Here's how the part is built. I have some questions about the finished solid (model axes, mm). Face numbers are marked on the shaded views. A direction names the side the tool comes from. Coordinates: 2 decimals unless noted, no trailing zeros. Write each loop counter-clockwise with the first axis right and the second up, starting at its lowest first coordinate (ties: lowest second). Pieces come first, ordered by that corner, then holes. Notation, with made-up numbers: (72, 34.25) -> (117, 34.25) arc R33 ccw to (117, 72.25) -> close; hole circle Ø8 at (36, 0). An arc over 180 degrees is marked (long way). Put each result on its own line as item: value. Start each with the question number.
Item 1: I need wall thicknesses on line 1 (X direction, y = -5, z = -2); line 2 (X direction, y = 11, z = -10); line 3 (X direction, y = -10, z = -11.5). Which ranges of each line are inside material? Lowest first, please. Write a range as [from, to].
Item 2: If we mould it in two halves opening along X, with no side actions, what happens to the marked faces 6, 7, 8 and 9? For each: released by +X, released by -X, zero draft, split by the parting line, or undercut.
Item 3: I want a section at A-A, the plane y = -4. List the corners of the cut face in (x, z) for me, then the cut area to 3 significant figures.
Item 4: I want a section at B-B, the plane z = -11. State how many separate pieces and enclosed holes the cut face has, then the cut area to 3 significant figures.
Item 5: For pin 1 (2 mm diameter, centred on x = -9.5, z = -8.5, fed in from +Y); pin 2 (1 mm diameter, centred on x = -14.5, z = -5.5, fed in from +Y); pin 3 (3.5 mm diameter, centred on y = 13, z = -10.5, fed in from -X), each with a flat end and sliding along its axis, tell me the tip position at first contact or that it passes through.
Item 6: I want a section at C-C, the plane x = -27. List the corners of the cut face in (y, z) for me.
Item 7: On a 3-axis mill with a long thin cutter (end or side, diameter ignored), from which of +Z, -Z, +X, -X, +Y, -Y can I reach the whole of each face in a straight line? I mean the marked faces 1, 2, 3, 4 and 5. Say none if no direction works.
from build123d import *

# Parameters (mm, degrees)
F0_W     = 6.6796690226
F0_H     = 6.4269647701
F0_W_2   = 4.7415380832
F0_H_2   = 6.6773667932
F0_W_3   = 4.3679763669
F0_H_3   = 6.5104326932
F3_DEPTH = 17.91377


# Not quite as in the source:
# - a feature of the source that left no trace in its solid (it failed there, or was rolled back) is left out


with BuildPart() as f3:
    # F0 (on Top) → F3 (new body)
    with BuildSketch(Plane.XY):
        with BuildLine():
            Line((-7.7901906334, 10.6832636405), (-7.7901906334, 8.2267736901))
            Line((-7.7901906334, 8.2267736901), (-7.7901906334, 1.7163409969))
            Line((-7.7901906334, 1.7163409969), (-7.7901906334, -5.3760232519))
            add(Edge.make_bspline(
                [(-7.7901906334, -5.3760232519), (-5.8573922142, -16.4409913238), (6.3671558164, -13.6890839785), (6.6410573199, -5.3240084089)],
                knots=[0, 0, 0, 0, 14.4313416921, 14.4313416921, 14.4313416921, 14.4313416921], degree=3))
            Line((6.6410573199, -5.3240084089), (6.6410573199, 1.7169426428))
            Line((6.6410573199, 1.7169426428), (6.6410573199, 8.1439074129))
            Line((6.6410573199, 8.1439074129), (6.6410573199, 10.5028618127))
            add(Edge.make_bspline(
                [(-7.7901906334, 10.6832636405), (-7.9460730776, 20.2635042254), (6.0135321692, 21.5757451952), (6.6410573199, 10.5028618127)],
                knots=[0, 0, 0, 0, 14.4323754909, 14.4323754909, 14.4323754909, 14.4323754909], degree=3))
        make_face()
        with BuildLine():
            Line((-3.0246356037, 8.227375336), (-3.0246356037, 10.4858698323))
            add(Edge.make_bspline(
                [(-3.0246356037, 10.4858698323), (-2.9879831709, 15.9807316959), (2.4520969018, 14.104841277), (1.7169024795, 10.4636372998)],
                knots=[0, 0, 0, 0, 4.7415902058, 4.7415902058, 4.7415902058, 4.7415902058], degree=3))
            Line((1.7169024795, 10.4636372998), (1.7169024795, 8.227375336))
            Line((1.7169024795, 8.227375336), (1.7169024795, 1.5500085428))
            Line((1.7169024795, 1.5500085428), (1.7169024795, -5.1218802109))
            add(Edge.make_bspline(
                [(-3.0246356037, -5.2313073538), (-2.9015108012, -9.3426071107), (2.1988428198, -8.9745400473), (1.7169024795, -5.1218802109)],
                knots=[0, 0, 0, 0, 4.7428006171, 4.7428006171, 4.7428006171, 4.7428006171], degree=3))
            Line((-3.0246356037, -5.2313073538), (-3.0246356037, 1.5500085428))
            Line((-3.0246356037, 1.5500085428), (-3.0246356037, 8.227375336))
        make_face(mode=Mode.SUBTRACT)
        with BuildLine():
            add(Edge.make_bspline(
                [(-20.5391882093, 13.9101054404), (-15.6776210399, 14.6662937362), (-16.1226423563, 15.8139783774), (-15.4372690351, 17.8214814399)],
                knots=[0, 0, 0, 0, 6.4287200491, 6.4287200491, 6.4287200491, 6.4287200491], degree=3))
            Line((-20.5391882093, 13.9101054404), (-20.5391882093, 10.912990186))
            Line((-20.5391882093, 10.912990186), (-16.858519438, 10.912990186))
            Line((-16.858519438, 10.912990186), (-16.858519438, 8.1935095558))
            Line((-16.858519438, 8.1935095558), (-16.858519438, 1.6338703002))
            Line((-16.858519438, 1.6338703002), (-16.858519438, -11.9715025764))
            Line((-16.858519438, -11.9715025764), (-12.1581670002, -11.9715025764))
            Line((-12.1581670002, -11.9715025764), (-12.1581670002, 1.7163409969))
            Line((-12.1581670002, 1.7163409969), (-12.1581670002, 8.2267736901))
            Line((-12.1581670002, 8.2267736901), (-12.1581670002, 17.8214814399))
            Line((-12.1581670002, 17.8214814399), (-15.4372690351, 17.8214814399))
        make_face()
        with BuildLine():
            Line((13.3207263425, 10.6080584228), (13.3207263425, 8.1439074129))
            Line((13.3207263425, 8.1439074129), (13.3207263425, 1.7169426428))
            Line((13.3207263425, 1.7169426428), (13.3207263425, -11.9709009305))
            Line((13.3207263425, -11.9709009305), (17.8177803755, -11.9709009305))
            Line((17.8177803755, -11.9709009305), (17.8177803755, 1.7169426428))
            Line((17.8177803755, 1.7169426428), (17.8177803755, 8.227375336))
            Line((17.8177803755, 8.227375336), (17.8177803755, 17.8220830858))
            Line((17.8177803755, 17.8220830858), (15.0071214885, 17.8220830858))
            add(Edge.make_bspline(
                [(9.5731783658, 13.6997830123), (14.1142597422, 14.0927145258), (14.2135191709, 16.0034615546), (15.0071214885, 17.8220830858)],
                knots=[0, 0, 0, 0, 6.820637489, 6.820637489, 6.820637489, 6.820637489], degree=3))
            Line((9.5731783658, 13.6997830123), (9.5731783658, 10.6080584228))
            Line((9.5731783658, 10.6080584228), (13.3207263425, 10.6080584228))
        make_face()
        with BuildLine():
            Line((-16.858519438, 1.6338703002), (-16.858519438, 8.1935095558))
            Line((-16.858519438, 8.1935095558), (-32.2274787855, 8.1935095558))
            add(Edge.make_bspline(
                [(-32.2274787855, 8.1935095558), (-32.5451358574, 5.8624682682), (-32.6565323778, 3.6785873351), (-32.5981434394, 1.6338703002)],
                knots=[2.9954620198, 2.9954620198, 2.9954620198, 2.9954620198, 7.0566986479, 7.0566986479, 7.0566986479, 7.0566986479], degree=3))
            Line((-32.5981434394, 1.6338703002), (-16.858519438, 1.6338703002))
        make_face()
        with BuildLine():
            Line((17.8177803755, 1.7169426428), (32.925114671, 1.7169426428))
            add(Edge.make_bspline(
                [(32.925114671, 1.7169426428), (32.9640628967, 4.0950280506), (32.7178774406, 6.2881527237), (32.3742319383, 8.227375336)],
                knots=[25.2691995487, 25.2691995487, 25.2691995487, 25.2691995487, 32.9729040179, 32.9729040179, 32.9729040179, 32.9729040179], degree=3))
            Line((32.3742319383, 8.227375336), (17.8177803755, 8.227375336))
            Line((17.8177803755, 8.227375336), (17.8177803755, 1.7169426428))
        make_face()
        with Locations((9.9808918312, 4.9304250279)):
            Rectangle(F0_W, F0_H)
        with Locations((-0.6538665621, 4.8886919394)):
            Rectangle(F0_W_2, F0_H_2)
        with Locations((-9.9741788168, 4.9715573435)):
            Rectangle(F0_W_3, F0_H_3)
    extrude(amount=-F3_DEPTH)


solid = f3.part
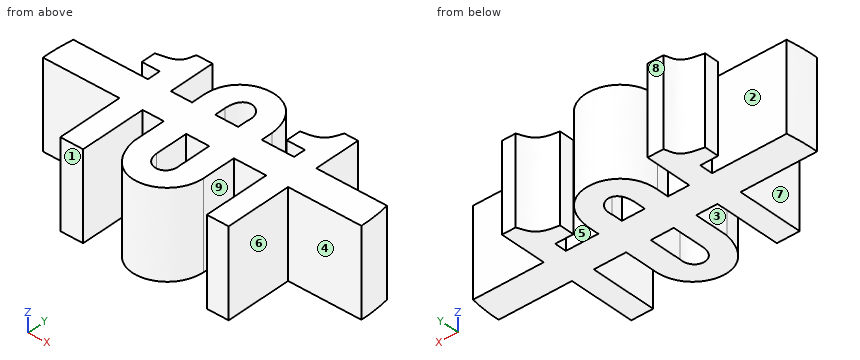
Calculated:
1. line 1: x = [-16.86, -12.16], [-7.79, -3.02], [1.72, 6.64], [13.32, 17.82]
1. line 2: x = [-20.54, -12.16], [-7.79, -3], [1.78, 6.6], [9.57, 17.82]
1. line 3: x = [-16.86, -12.16], [-5.92, 4.91], [13.32, 17.82]
2. face 6: released by +X
2. face 7: released by -X
2. face 8: zero draft
2. face 9: undercut
3. outline: (-16.86, -17.91) -> (-12.16, -17.91) -> (-12.16, 0) -> (-16.86, 0) -> close; (-7.79, -17.91) -> (-3.02, -17.91) -> (-3.02, 0) -> (-7.79, 0) -> close; (1.72, -17.91) -> (6.64, -17.91) -> (6.64, 0) -> (1.72, 0) -> close; (13.32, -17.91) -> (17.82, -17.91) -> (17.82, 0) -> (13.32, 0) -> close
3. area: 338 mm2
4. separate pieces: 1
4. enclosed holes: 2
4. area: 898 mm2
5. pin 1: stops at y = 8.23
5. pin 2: stops at y = 17.82
5. pin 3: stops at x = -20.54
6. outline: (1.63, -17.91) -> (8.19, -17.91) -> (8.19, 0) -> (1.63, 0) -> close
7. face 1: +Z, -Z, -X, -Y
7. face 2: +Z, -Z, -X
7. face 3: +Z, -Z, -Y
7. face 4: +Z, -Z, +X, -Y
7. face 5: +Z, -Z
